from build123d import *

# Parameters (mm, degrees)
SKETCH039_R           = 14.5
PAD016_DEPTH          = 5
POCKET022_DEPTH       = 2.5
SKETCH041_R           = 2
POCKET023_DEPTH       = 87.6327130405
POLARPATTERN001_COUNT = 3
SKETCH042_R           = 4.25
PAD017_DEPTH          = 1.5
POCKET024_DEPTH       = 5.001
POCKET024_DEPTH_BACK  = 1.501


with BuildPart() as part:
    # Sketch039 → Pad016 (new body)
    with BuildSketch(Plane.XY.offset(55.1)):
        Circle(SKETCH039_R)
    extrude(amount=PAD016_DEPTH)

    # Sketch040 → Pocket022 (cut)
    with BuildSketch(Plane.XY.offset(60.1)):
        with BuildLine():
            Line((-14.4052301376, 1.6550965782), (-8.5148861812, 2.4215481911))
            Line((-8.5148861812, 2.4215481911), (-6.1481704596, -0.8))
            Line((-6.1481704596, -0.8), (-7.6116603747, -4.5199345858))
            Line((-7.6116603747, -4.5199345858), (-13.5020043311, -5.2863861987))
            ThreePointArc((-14.4052301376, 1.6550965782), (-14.3787857522, -1.8709677419), (-13.5020043311, -5.2863861987))
        make_face()
    pocket022 = extrude(amount=-POCKET022_DEPTH, mode=Mode.SUBTRACT)

    # Sketch041 → Pocket023 (cut, through all)
    with BuildSketch(Plane.XY.offset(55.1)):
        with Locations((-10.0992623493, -1.43)):
            Circle(SKETCH041_R)
    pocket023 = extrude(amount=POCKET023_DEPTH, mode=Mode.SUBTRACT)

    # PolarPattern001: Pocket023, Pocket022 ×3 about axis
    polarpattern001_axis = Axis((0, 0, 55.1), (0, 0, 1))
    for i in range(1, POLARPATTERN001_COUNT):
        add(pocket023.rotate(polarpattern001_axis, i * 360 / POLARPATTERN001_COUNT), mode=Mode.SUBTRACT)
        add(pocket022.rotate(polarpattern001_axis, i * 360 / POLARPATTERN001_COUNT), mode=Mode.SUBTRACT)

    # Sketch042 → Pad017 (join)
    with BuildSketch(Plane.XY.offset(60.1)):
        Circle(SKETCH042_R)
    extrude(amount=PAD017_DEPTH)

    # Sketch043 → Pocket024 (cut, two sides)
    with BuildSketch(Plane.XY.offset(60.1)) as pocket024_sk:
        with BuildLine():
            Line((2, 1.5), (2, -1.5))
            ThreePointArc((2, 1.5), (-2.5, 0), (2, -1.5))
        make_face()
    extrude(amount=-POCKET024_DEPTH, mode=Mode.SUBTRACT)
    extrude(pocket024_sk.sketch, amount=POCKET024_DEPTH_BACK, mode=Mode.SUBTRACT)


solid = part.part
Build history of the part. All positions in model axes, mm. A direction names the side the tool comes from. Coordinates: 2 decimals unless noted, no trailing zeros. Order: outer loops, then holes, each group sorted by start corner. A loop starts at its lowest first (then second) coordinate and runs counter-clockwise, first axis right, second up. Notation, with made-up numbers: (4.25, 86) - (29.25, 86) arc R20 cw to (29.25, 122) - close; hole circle Ø8 at (-31, 85.5). An arc over 180 degrees is marked (long way). Write item = value, one per line. Start each with the question number.
1) Saw through at B-B on y = 9.5. Write the cut outline in (x, z), then the cut area to 3 significant figures.
2) Saw through at D-D on z = 56. Write the cut outline in (x, y).
3) Saw through at C-C on y = 0. Write the cut outline in (x, z).
4) Saw through at A-A on z = 58. Write the cut outline in (x, y), then the cut area to 3 significant figures.
5) 3-axis set-ups, long thin cutter, end or side, ignore diameter. For faces 4 (the face through (2, 0, 58)), 5 (the face through (9.5, -6.66, 58.87)), 6 (the face through (5.72, -4.63, 58.87)): which of +Z, -Z, +X, -X, +Y, -Y reach the whole face in a straight line?
6) Two-plate mould, pull along X, no slides. Class faces 1 (the face through (6, 11, 57.6)), 2 (the face through (-3.143, -14.155, 57.565)), 3 (the face through (3, 0, 55.1)): pulls with the +X half, pulls with the -X half, needs draft (parallel to the pull), parting line crosses it, or undercut.
7) Flat gauge pins, fed straight in: pin 1 Ø1 at (x, z) = (2, 58) entering from +Y; pin 2 Ø4.5 at (x, y) = (5.5, 11) entering from +Z; pin 3 Ø3 at (x, y) = (-10.1, -1.43) entering from +Z; pin 4 Ø7 at (x, y) = (8.5, -8.5) entering from +Z. Where does each tip first touch, or does it go through?
8) Wall check: line 1 along Z through (x, y) = (4, 6.75); line 2 along Z through (x, y) = (5.5, 0); line 3 along X through (y, z) = (11.5, 59). Give the ranges that are in metal, low to high. Write a range as from..to.
From the geometry:
q1.outline = (-10.95, 55.1) - (1.81, 55.1) - (1.81, 57.6) - (0.16, 57.6) - (0.16, 60.1) - (-10.95, 60.1) - close; (5.81, 55.1) - (10.95, 55.1) - (10.95, 60.1) - (7.74, 60.1) - (7.74, 57.6) - (5.81, 57.6) - close
q1.area = 80.6 mm^2
q2.outline = circle Ø29 at (0, 0); hole circle Ø4 at (-10.1, -1.43); hole circle Ø4 at (3.81, 9.46); hole (2, -1.5) - (2, 1.5) arc R2.5 ccw (long way) to start; hole circle Ø4 at (6.29, -8.03)
q3.outline = (-14.5, 55.1) - (-11.5, 55.1) - (-11.5, 57.6) - (-14.5, 57.6) - close; (-8.7, 55.1) - (-2.5, 55.1) - (-2.5, 61.6) - (-4.25, 61.6) - (-4.25, 60.1) - (-6.74, 60.1) - (-6.74, 57.6) - (-8.7, 57.6) - close; (2, 55.1) - (14.5, 55.1) - (14.5, 60.1) - (4.25, 60.1) - (4.25, 61.6) - (2, 61.6) - close
q4.outline = (-14.41, 1.66) - (-8.51, 2.42) - (-6.15, -0.8) - (-7.61, -4.52) - (-13.5, -5.29) arc R14.5 ccw to (5.77, -13.3) - (2.16, -8.58) - (3.77, -4.92) - (7.72, -4.33) - (11.33, -9.05) arc R14.5 ccw to (8.64, 11.65) - (6.35, 6.16) - (2.38, 5.72) - (-0.11, 8.85) - (2.17, 14.34) arc R14.5 ccw to start; hole (2, -1.5) - (2, 1.5) arc R2.5 ccw (long way) to start
q4.area = 491 mm^2
q5.face_4 = +Z, -Z
q5.face_5 = +Z, -Y
q5.face_6 = +Z
q6.face_1 = undercut
q6.face_2 = parting line crosses it
q6.face_3 = needs draft
q7.pin_1 = 14.42
q7.pin_2 = 57.6
q7.pin_3 = through
q7.pin_4 = 60.1
q8.line_1 = 55.1..57.6
q8.line_2 = 55.1..60.1
q8.line_3 = -8.83..0.99, 8.57..8.83
